Design review of the part built by this model. Coordinates are the model's own, in mm. A direction names the side the tool comes from. Coordinates: 2 decimals unless noted, no trailing zeros. Write each loop counter-clockwise with the first axis right and the second up, starting at its lowest first coordinate (ties: lowest second). Pieces come first, ordered by that corner, then holes.
Q1. To check wall thickness, follow probe 1 along X at (y, z) = (303, 12.25); probe 2 along Y at (x, z) = (107, 7.5); probe 3 along X at (y, z) = (249, 8.5). State the ranges of each line that lie inside material, in increasing order.
Q2. Add section B-B, the plane y = 163. Give the boundary of the cut face in (x, z), plus the area to 3 significant figures.
Q3. The part is to be moulded in two halves that separate along X. For faces 4 (the face through (24, 331.193, 9)), 5 (the face through (84, 313.193, 9)), 6 (the face through (119.168, 178.935, 8.874)), say which applies: +X half, -X half, draft (parallel to the pull), parting line (faces both ways), or undercut.
Q4. Machinability: for faces 1 (the face through (166.876, 315, 9)), 2 (the face through (116.876, 322, 9)), 3 (the face through (-0.551, 321, 9)), which of the approach directions +Z, -Z, +X, -X, +Y, -Y give a long, thin tool a straight path to every point of the face, cutting with its end or side? Answer none if there is none.
Q5. Add section C-C, the plane x = 57.5. Give the boundary of the cut face in (y, z).
Q6. Clearance check with flat-ended pins moving along their axes: pin 1 Ø5.5 at (y, z) = (316, 8.5) entering from +X; pin 2 Ø1.5 at (x, z) = (39.5, 10) entering from -Y; pin 3 Ø6 at (y, z) = (170.5, 11) entering from -X. State where each tip first meets the part, or that it passes through.
Q7. Add section A-A, the plane z = 14.75. Give the boundary of the cut face in (x, y).
Autodesk Inventor part; units mm, degrees
ref_plane "YZ Plane" through (0, 0, 0) normal (1, 0, 0) x (0, 1, 0)
ref_plane "XZ Plane" through (0, 0, 0) normal (0, 1, 0) x (-1, 0, 0)
ref_plane "XY Plane" through (0, 0, 0) normal (0, 0, 1) x (1, 0, 0)
sketch "Sketch1" plane through (0, 0, 0) normal (0, 0, 1) x (1, 0, 0)
  arc A0 (176.5598, 33.6793) -> (12.6136, 287.2326) centre (-204.4335, -32.8889) ccw
  line L0 (167.9834, 291.8121) -> (218.9792, 109.3407)
  arc A1 (227.759, 27.1192) -> (218.9792, 109.3407) centre (-21.7947, 42.0509) ccw
  arc A2 (207.2823, -0.2492) -> (227.2466, 18.5563) centre (207.2823, 19.7508) ccw
  arc A3 (176.5598, 33.6793) -> (189.5473, 6.5592) centre (231.3648, 43.255) ccw
  arc A4 (189.5473, 6.5592) -> (204.58, -0.2492) centre (204.58, 19.7508) ccw
  line L1 (207.2823, -0.2492) -> (204.58, -0.2492)
  line L2 (227.759, 27.1192) -> (227.2466, 18.5563)
  arc A5 (248.2588, 303.6927) -> (197.3635, 355.4189) centre (196.5258, 303.6927) ccw
  line L3 (248.2588, 303.6927) -> (248.2588, 286.4547)
  arc A6 (222.3411, 252.6536) -> (248.2588, 286.4547) centre (213.2588, 286.4547) ccw
  line L4 (-281.6446, 363.1761) -> (197.3635, 355.4189)
  arc A7 (222.3411, 252.6536) -> (-337.0597, 3.3874) centre (731.561, -1642.4666) ccw
  line L5 (297.4263, 347.2322) -> (-473.2183, 347.2322) construction
  line L6 (-303.5209, 267.588) -> (-100.5419, 267.588)
  line L7 (-94.1908, 238.9989) -> (-285.5647, 149.5573)
  arc A8 (-94.1908, 238.9989) -> (-100.5419, 267.588) centre (-100.5419, 252.588) ccw
  arc A9 (-316.1527, 274.4986) -> (-303.5209, 267.588) centre (-303.5209, 282.588) ccw
  line L8 (-324.4601, 363.1761) -> (-281.6446, 363.1761)
  line L9 (-353.5533, 332.9002) -> (-316.1527, 274.4986)
  arc A10 (-324.4601, 363.1761) -> (-354.3192, 336.0808) centre (-324.4601, 333.1761) ccw
  arc A11 (-354.3192, 336.0808) -> (-353.5533, 332.9002) centre (-349.3427, 335.5967) ccw
  arc A12 (-358.3707, 23.1982) -> (-337.0597, 3.3874) centre (-345.2282, 15.9682) ccw
  line L10 (-292.3562, 143.1982) -> (-358.3707, 23.1982)
  arc A13 (-285.5647, 149.5573) -> (-292.3562, 143.1982) centre (-279.2137, 135.9682) ccw
  line L11 (-280.0505, 115.5231) -> (-264.2795, 106.8471)
  line L12 (-288.3795, 63.0385) -> (-264.2795, 106.8471)
  line L13 (-304.1505, 71.7145) -> (-288.3795, 63.0385)
  line L14 (-304.1505, 71.7145) -> (-280.0505, 115.5231)
  line L15 (-300.243, 286.193) -> (-282.243, 286.193)
  line L16 (-282.243, 336.193) -> (-300.243, 336.193)
  line L17 (-300.243, 336.193) -> (-300.243, 286.193)
  line L18 (199.757, 276.193) -> (181.757, 276.193)
  line L19 (181.757, 276.193) -> (181.757, 336.193)
  line L20 (181.757, 336.193) -> (199.757, 336.193)
  line L21 (199.757, 336.193) -> (199.757, 276.193)
  line L22 (-350.0834, 336.193) -> (288.2929, 336.193) construction
  line L23 (-282.243, 286.193) -> (-282.243, 336.193)
  line L24 (-194.243, 331.193) -> (-194.243, 313.193)
  line L25 (-94.243, 331.193) -> (-94.243, 313.193)
  line L26 (-194.243, 331.193) -> (-94.243, 331.193)
  line L27 (-94.243, 313.193) -> (-194.243, 313.193)
  line L28 (-282.243, 346.193) -> (-282.243, 276.193)
  line L29 (-282.243, 313.193) -> (-282.243, 331.193)
  line L30 (-282.243, 276.193) -> (-300.243, 276.193)
  line L31 (-300.243, 276.193) -> (-300.243, 346.193)
  line L32 (-300.243, 346.193) -> (-282.243, 346.193)
  line L33 (-6.243, 331.193) -> (-6.243, 313.193)
  line L34 (-6.243, 331.193) -> (93.757, 331.193)
  line L35 (93.757, 313.193) -> (-6.243, 313.193)
  line L36 (93.757, 331.193) -> (93.757, 313.193)
  line L37 (181.757, 331.193) -> (181.757, 313.193)
  line L38 (181.757, 346.193) -> (181.757, 266.193)
  line L39 (199.757, 346.193) -> (181.757, 346.193)
  line L40 (181.757, 266.193) -> (199.757, 266.193)
  line L41 (199.757, 266.193) -> (199.757, 346.193)
  line L42 (-0.5508, 312.0632) -> (-0.5508, 313.193)
  line L43 (166.8762, 299.8869) -> (166.8762, 313.193)
  line L44 (166.8762, 313.193) -> (-0.5508, 313.193)
  line L45 (166.8762, 313.193) -> (166.8762, 331.193)
  line L46 (166.8762, 331.193) -> (116.8762, 331.193)
  line L47 (116.8762, 331.193) -> (116.8762, 313.193)
  line L48 (-0.5508, 313.193) -> (-0.5508, 331.193)
  line L49 (-0.5508, 331.193) -> (49.4492, 331.193)
  line L50 (49.4492, 331.193) -> (49.4492, 313.193)
  arc A14 (-0.5508, 312.0632) -> (12.6136, 287.2326) centre (29.4492, 312.0632) ccw
  arc A15 (166.8762, 299.8869) -> (167.9834, 291.8121) centre (196.8762, 299.8869) ccw
  point P0 (0, 0)
  point P1 (-0.5508, 295.7736)
  point P2 (166.8762, 295.7736)
  point P3 (263.5097, 263.2389)
  point P4 (-311.7271, 267.588)
  point P5 (-289.9977, 147.4855)
  point P6 (-388.1512, -30.9362)
  point P7 (-291.243, 346.193)
  point P8 (372.0119, 346.193)
  dimension "d0" = 20
  dimension "d1" = 250
  dimension "d32" = 15
  dimension "d33" = 35
  dimension "d34" = 120
  dimension "d35" = 30
  dimension "d36" = 5
  dimension "d37" = 50
  dimension "d38" = 60
  dimension "d39" = 18
  dimension "d40" = 500
  dimension "d41" = 70
  dimension "d42" = 80
  dimension "d43" = 18
  dimension "d44" = 464
  dimension "d45" = 100
  dimension "d46" = 100
  dimension "d47" = 88
  dimension "d48" = 88
  dimension "d49" = 50
  dimension "d50" = 50
  dimension "d51" = 30
  dimension "d52" = 5.6922
  dimension "d53" = 67.427
  dimension "d54" = 30
extrude "Extrusion1" add sketch "Sketch1" along normal blind 18 contours A0 A7 L0 A1 L2 A2 L1 A4 A3 | A0 A14 L42 L35 L44 L43 A15 L0 A7
sketch "Sketch7" plane through (0, 0, 18) normal (0, 0, 1) x (1, 0, 0)
  line L0 (166.8762, 313.193) -> (166.8762, 331.193)
  line L1 (166.8762, 331.193) -> (116.8762, 331.193)
  line L2 (116.8762, 331.193) -> (116.8762, 313.193)
  line L3 (-0.5508, 313.193) -> (-0.5508, 331.193)
  line L4 (-0.5508, 331.193) -> (49.4492, 331.193)
  line L5 (49.4492, 331.193) -> (49.4492, 313.193)
  line L6 (166.8762, 313.193) -> (116.8762, 313.193)
  line L7 (49.4492, 313.193) -> (-0.5508, 313.193)
  point P0 (0, 0)
  dimension "d67" = 50
  dimension "d68" = 50
  dimension "d69" = 67.427
extrude "Extrusion5" add sketch "Sketch7" against normal blind 18
sketch "Sketch8" plane through (0, 0, 18) normal (0, 0, 1) x (1, 0, 0)
  line L0 (195.4129, 0.9342) -> (223.5969, 0.9342)
  line L1 (223.5969, 0.9342) -> (223.5969, -9.3542)
  line L2 (223.5969, -9.3542) -> (195.4129, -9.3542)
  line L3 (195.4129, -9.3542) -> (195.4129, 0.9342)
  point P0 (0, 0)
extrude "Extrusion6" cut sketch "Sketch8" against normal blind 18
properties part number "Pata" material "Wood (Birch)"
Here are the results:
1. probe 1: x = 0.85 to 166.88
1. probe 2: y = 196.45 to 313.19
1. probe 3: x = 60.38 to 179.95
2. outline: (129.06, 0) - (203.98, 0) - (203.98, 18) - (129.06, 18) - close
2. area: 1,350 mm2
3. face 4: draft
3. face 5: undercut
3. face 6: -X half
4. face 1: +Z, -Z, +X, +Y
4. face 2: +Z, -Z, +Y
4. face 3: +Z, -Z, -X, +Y, -Y
5. outline: (251.68, 0) - (313.19, 0) - (313.19, 18) - (251.68, 18) - close
6. pin 1: stops at x = 166.88
6. pin 2: stops at y = 266.64
6. pin 3: stops at x = 122.66
7. outline: (-0.55, 312.06) arc R30 ccw to (12.61, 287.23) arc R386.77 cw to (176.56, 33.68) arc R55.64 ccw to (189.55, 6.56) arc R20 ccw to (197.8, 0.93) - (214.06, 0.93) arc R20 ccw to (227.25, 18.56) - (227.76, 27.12) arc R250 ccw to (218.98, 109.34) - (167.98, 291.81) arc R30 cw to (166.88, 299.89) - (166.88, 331.19) - (116.88, 331.19) - (116.88, 313.19) - (49.45, 313.19) - (49.45, 331.19) - (-0.55, 331.19) - close
